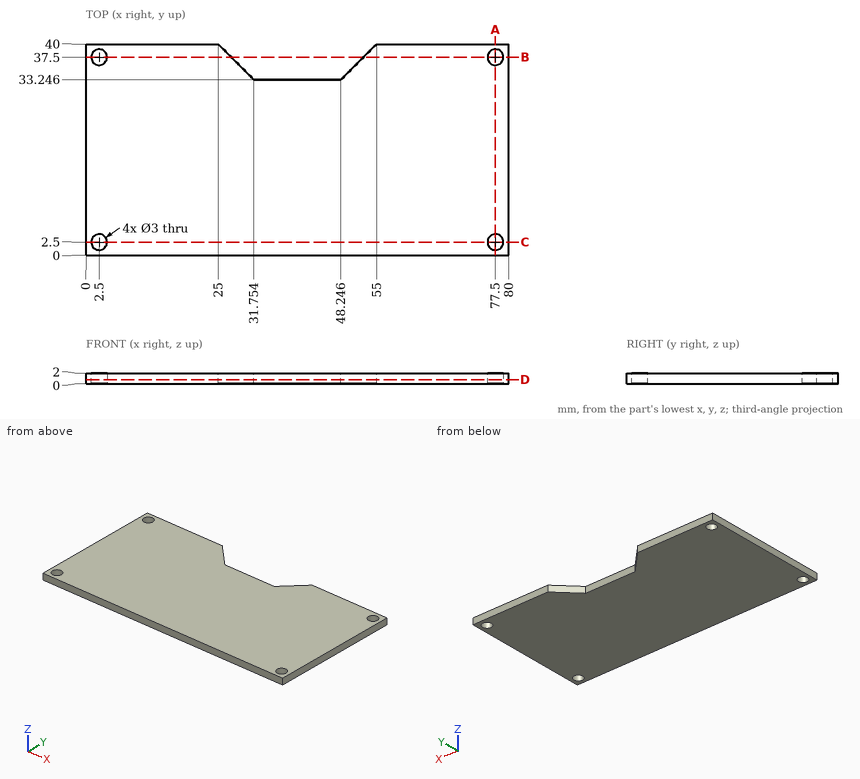
Print and shaded views of the part. All mm, measured from the part's lowest x, y and z. Give positions to 0.01 mm unless a question says otherwise; leave off trailing zeros. Loops run counter-clockwise (first coordinate to the right, second up) from the corner with the lowest first, then second, coordinate; pieces in that order, holes last. Notation, with made-up numbers: M -25,-38 L 29,-38 A20 ccw 29,-33 Z; hole C 1,47 d7. An arc over 180 degrees is marked long. Write each question's results on one line, items separated by ' | '.
Q1. Band-saw the part on A-A on x = 77.5. Write the cut outline in (y, z), and give its area (3 significant figures).
Geometry check:
outline: M 0,0 L 1,0 L 1,2 L 0,2 Z; M 4,0 L 36,0 L 36,2 L 4,2 Z; M 39,0 L 40,0 L 40,2 L 39,2 Z | area: 68.0 mm²
Q2. Flat gauge pins, fed straight in: P1, Ø1, axis at x = 42, z = 1, coming from the +Y side; P2, Ø1.8, axis at x = 77.5, y = 37.5, coming from the -Z side. Where does each tip first touch, or does it go through?
Geometry check:
P1: stops at y = 33.25 | P2: passes through
Q3. Band-saw the part on D-D on z = 0.8. Write the cut outline in (x, y), and give its area (3 significant figures).
Geometry check:
outline: M 0,0 L 80,0 L 80,40 L 55,40 L 48.25,33.25 L 31.75,33.25 L 25,40 L 0,40 Z; hole C 2.5,2.5 d3; hole C 2.5,37.5 d3; hole C 77.5,2.5 d3; hole C 77.5,37.5 d3 | area: 3,010 mm²
Q4. Band-saw the part on C-C on y = 2.5. Write the cut outline in (x, z), and give its area (3 significant figures).
Geometry check:
outline: M 0,0 L 1,0 L 1,2 L 0,2 Z; M 4,0 L 76,0 L 76,2 L 4,2 Z; M 79,0 L 80,0 L 80,2 L 79,2 Z | area: 148 mm²
Q5. Band-saw the part on B-B on y = 37.5. Write the cut outline in (x, z).
Geometry check:
outline: M 0,0 L 1,0 L 1,2 L 0,2 Z; M 4,0 L 27.5,0 L 27.5,2 L 4,2 Z; M 52.5,0 L 76,0 L 76,2 L 52.5,2 Z; M 79,0 L 80,0 L 80,2 L 79,2 Z
Q6. Probe probe 1 along Y at (x, z) = (2.5, 0.5); probe 2 along Y at (x, z) = (29, 1.1); probe 3 along X at (y, z) = (3, 1.35) (1 decimal). List the from-to ranges inside material, lowest first.
Geometry check:
probe 1: y = 0 to 1, 4 to 36, 39 to 40 | probe 2: y = 0 to 36 | probe 3: x = 0 to 1.1, 3.9 to 76.1, 78.9 to 80
